Here's how the part is built. I have some questions about the finished solid (model axes, mm). Face numbers are marked on the shaded views. A direction names the side the tool comes from. Give positions to 0.01 mm unless a question says otherwise; leave off trailing zeros. Write each loop counter-clockwise with the first axis right and the second up, starting at its lowest first coordinate (ties: lowest second). Pieces come first, ordered by that corner, then holes. Notation, with made-up numbers: (-17, 1) - (26, 1) arc R32 cw to (26, 40) - close; hole circle Ø11 at (-32, 33). An arc over 180 degrees is marked (long way). One line per item, written item: value. Start each with the question number.
1) On a 3-axis mill with a long thin cutter (end or side, diameter ignored), from which of +Z, -Z, +X, -X, +Y, -Y can I reach the whole of each face in a straight line? I mean the marked faces 1, 2 and 3. Say none if no direction works.
2) Please list where these lines run through material, in increasing order: L1, parallel to Y at x = -2.75, z = -5; L2, parallel to Z at x = -4, y = 12.75 (3 decimals); L3, parallel to Y at x = 3, z = 2.5. Write a range as [from, to].
3) I'm going to push flat-ended pins straight in: P1, Ø3, axis at x = -6.5, z = -1, coming from the +Y side; P2, Ø5.5, axis at y = 16, z = -0.5, coming from the -X side. Where does each tip first touch, or does it pass through?
4) Imagine slicing it at A-A on x = 8.25. Write out the boundary of the cut face in (y, z), plus the area to 3 significant figures.
5) Imagine slicing it at B-B on z = -5. Write out the boundary of the cut face in (x, y), plus the area to 3 significant figures.
from build123d import *

# Parameters (mm, degrees)
SKETCH1_W           = 20.32
SKETCH1_H           = 12.7
BOSS_EXTRUDE1_DEPTH = 12.7
BOSS_EXTRUDE2_DEPTH = 4.445


with BuildPart() as part:
    # Sketch1 → Boss-Extrude1 (new body)
    with BuildSketch(Plane(origin=(0, 0, 0), x_dir=(1, 0, 0), z_dir=(0, 1, 0))):
        Rectangle(SKETCH1_W, SKETCH1_H)
    extrude(amount=BOSS_EXTRUDE1_DEPTH)

    # Sketch2 → Boss-Extrude2 (add, symmetric)
    with BuildSketch(Plane.XY):
        with BuildLine():
            Line((-7.555612539, 17.803216518), (-7.555612539, 12.7))
            Line((-7.555612539, 12.7), (6.347718594, 12.7))
            add(Edge.make_bspline(
                [(-7.555612539, 17.803216518), (-1.024019713, 12.888036176), (6.347718594, 12.7)],
                knots=[0, 0, 0, 0.926306801, 0.926306801, 0.926306801], degree=2))
        make_face()
    extrude(amount=BOSS_EXTRUDE2_DEPTH, both=True)


solid = part.part
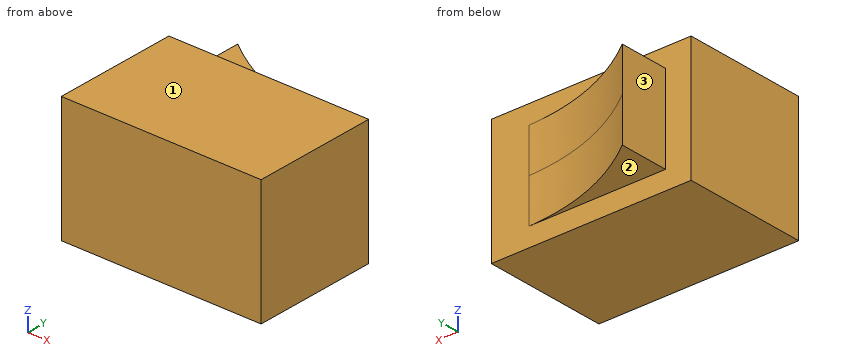
Numbers:
1. face 1: +Z, +X, -X, +Y, -Y
1. face 2: -Z, +X, -X, +Y
1. face 3: +Z, -Z, -X, +Y
2. L1: [0, 12.7]
2. L2: [-4.445, 4.445]
2. L3: [0, 13.04]
3. P1: y = 17.8
3. P2: x = -7.56
4. outline: (0, -6.35) - (12.7, -6.35) - (12.7, 6.35) - (0, 6.35) - close
4. area: 161 mm^2
5. outline: (-10.16, 0) - (10.16, 0) - (10.16, 12.7) - (-10.16, 12.7) - close
5. area: 258 mm^2
